Check sheet for the modelled part. Datum: model origin and axes. Units: mm. Coordinates: 2 decimals unless noted, no trailing zeros. Write each loop counter-clockwise with the first axis right and the second up, starting at its lowest first coordinate (ties: lowest second). Pieces come first, ordered by that corner, then holes. Notation, with made-up numbers: (-21.75, -34) - (-16.75, -34) arc R16 ccw to (-16.75, -22) - close; hole circle Ø11 at (89.5, -11). An arc over 180 degrees is marked (long way). Write each question's results on one line, items separated by ' | '.
from build123d import *

# Parameters (mm, degrees)
SKETCH_W          = 170
SKETCH_H          = 90
SKETCH_W_2        = 160
SKETCH_H_2        = 80
PAD_DEPTH         = 5
PAD001_DEPTH      = 5
PAD002_DEPTH      = 5
PAD003_DEPTH      = 5
SKETCH004_R       = 1.6
POCKET_DEPTH      = 5
SKETCH005_R       = 3
PAD004_DEPTH      = 3
SKETCH006_R       = 1.4
POCKET001_DEPTH   = 10
COPYSKETCH032_W   = 172
COPYSKETCH032_H   = 92
COPYSKETCH032_W_2 = 170
COPYSKETCH032_H_2 = 90
PAD006_DEPTH      = 5


with BuildPart() as part:
    # Sketch → Pad (new body)
    with BuildSketch(Plane.XY):
        Rectangle(SKETCH_W, SKETCH_H)
        Rectangle(SKETCH_W_2, SKETCH_H_2, mode=Mode.SUBTRACT)
    extrude(amount=PAD_DEPTH)

    # Sketch001 → Pad001 (join)
    with BuildSketch(Plane.XY):
        Polygon((-80, 40), (-80, 25), (-65, 40), align=None)
    extrude(amount=PAD001_DEPTH)

    # Sketch002 → Pad002 (join)
    with BuildSketch(Plane.XY):
        Polygon((-85, -45), (-75, -55), (-10, -55), (0, -45), align=None)
    extrude(amount=PAD002_DEPTH)

    # Sketch003 → Pad003 (join)
    with BuildSketch(Plane.XY):
        Polygon((0, 40), (-12, 30), (-22, 30), (-34, 40), align=None)
    extrude(amount=PAD003_DEPTH)

    # Sketch004 (on Face18 of Pad003) → Pocket (cut)
    with BuildSketch(Plane.XY.offset(5)):
        with Locations((-82.5, 42.5)):
            Circle(SKETCH004_R)
        with Locations((-82.5, -42.5)):
            Circle(SKETCH004_R)
        with Locations((82.5, -42.5)):
            Circle(SKETCH004_R)
        with Locations((82.5, 42.5)):
            Circle(SKETCH004_R)
    extrude(amount=-POCKET_DEPTH, mode=Mode.SUBTRACT)

    # Sketch005 (on Face18 of Pad003) → Pad004 (join)
    with BuildSketch(Plane.XY.offset(5)):
        with Locations((-75, 37.5)):
            Circle(SKETCH005_R)
        with Locations((-17, 37.5)):
            Circle(SKETCH005_R)
        with Locations((-75, -48.5)):
            Circle(SKETCH005_R)
        with Locations((-17, -48.5)):
            Circle(SKETCH005_R)
    extrude(amount=PAD004_DEPTH)

    # Sketch006 (on Face28 of Pad004) → Pocket001 (cut)
    with BuildSketch(Plane.XY.offset(8)):
        with Locations((-75, 37.5)):
            Circle(SKETCH006_R)
        with Locations((-17, 37.5)):
            Circle(SKETCH006_R)
        with Locations((-75, -48.5)):
            Circle(SKETCH006_R)
        with Locations((-17, -48.5)):
            Circle(SKETCH006_R)
    extrude(amount=-POCKET001_DEPTH, mode=Mode.SUBTRACT)

    # CopySketch032 → Pad006 (join)
    with BuildSketch(Plane.XY):
        Rectangle(COPYSKETCH032_W, COPYSKETCH032_H)
        Rectangle(COPYSKETCH032_W_2, COPYSKETCH032_H_2, mode=Mode.SUBTRACT)
    extrude(amount=PAD006_DEPTH)


solid = part.part
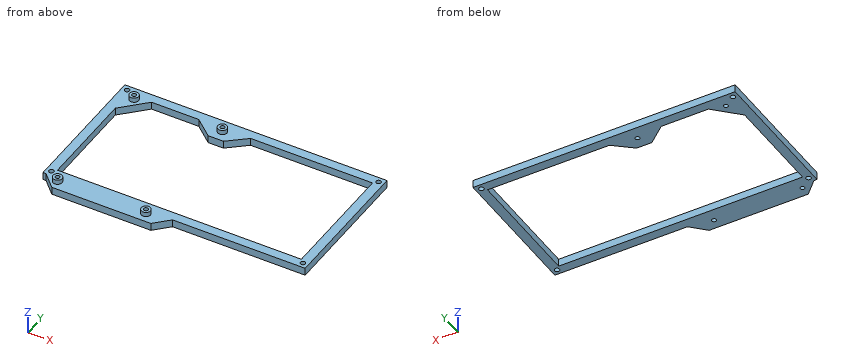
1. Go/stop test with flat-tipped pins: pin 1 (3 mm diameter, centred on x = 82.5, y = 42.5, fed in from -Z); pin 2 (3.5 mm diameter, centred on x = 82.5, y = -42.5, fed in from +Z); pin 3 (2.5 mm diameter, centred on x = 23, z = 1.5, fed in from -Y). Record where each tip stops, or that it passes through.
Values follow:
pin 1: passes through | pin 2: stops at z = 5 | pin 3: stops at y = -46
2. Sectioned sample at A-A (x = 82.5). Record the cut outline in (y, z), then the cut area to 3 significant figures.
Values follow:
outline: (-46, 0) - (-44.1, 0) - (-44.1, 5) - (-46, 5) - close; (-40.9, 0) - (40.9, 0) - (40.9, 5) - (-40.9, 5) - close; (44.1, 0) - (46, 0) - (46, 5) - (44.1, 5) - close | area: 428 mm^2
3. Material ranges on L1, parallel to Y at x = 82.5, z = 2.95; L2, parallel to Y at x = -75, z = 3.25; L3, parallel to Y at x = 24.5, z = 3.5, recorded low to high. Write a range as [from, to].
Values follow:
L1: y = [-46, -44.1], [-40.9, 40.9], [44.1, 46] | L2: y = [-55, -49.9], [-47.1, -40], [30, 36.1], [38.9, 46] | L3: y = [-46, -40], [40, 46]
4. Sectioned sample at B-B (y = -0.5). Record the cut outline in (x, z), then the cut area to 3 significant figures.
Values follow:
outline: (-86, 0) - (-80, 0) - (-80, 5) - (-86, 5) - close; (80, 0) - (86, 0) - (86, 5) - (80, 5) - close | area: 60.0 mm^2
5. Sectioned sample at D-D (y = 42.5). Record the cut outline in (x, z), then the cut area to 3 significant figures.
Values follow:
outline: (-86, 0) - (-84.1, 0) - (-84.1, 5) - (-86, 5) - close; (-80.9, 0) - (80.9, 0) - (80.9, 5) - (-80.9, 5) - close; (84.1, 0) - (86, 0) - (86, 5) - (84.1, 5) - close | area: 828 mm^2
6. Sectioned sample at C-C (x = -3). Record the cut outline in (y, z), then the cut area to 3 significant figures.
Values follow:
outline: (-48, 0) - (-40, 0) - (-40, 5) - (-48, 5) - close; (37.5, 0) - (46, 0) - (46, 5) - (37.5, 5) - close | area: 82.5 mm^2
